```python
from build123d import *

# Parameters (mm, degrees)
EXTRUDE_2_DEPTH        = 155
CHAMFER_1_SIZE         = 2
SKETCH_5_W             = 5.5
SKETCH_5_H             = 2.5
CUT_EXTRUDE_1_DEPTH    = 156.548424936
CUT_EXTRUDE_2_REACH    = 157.444
SKETCH_6_R             = 1.925
SKETCH_7_R             = 3.55
CUT_EXTRUDE_3_DEPTH    = 3.5
PATTERN_LINEAR_1_COUNT = 15
PATTERN_LINEAR_1_PITCH = 10
PATTERN_LINEAR_2_COUNT = 8
PATTERN_LINEAR_2_PITCH = 20


with BuildPart() as part:
    # 스케치4 → 보스-돌출2 (new body)
    with BuildSketch(Plane(origin=(0, 0, 0), x_dir=(0, 0, -1), z_dir=(1, 0, 0))):
        Polygon((0, 7.5), (0, -7.5), (-2.6, -7.5), (-5.25, -10.5), (-7.75, -8), (-7.75, 8), (-5.25, 10.5), (-2.6, 7.5), align=None)
    extrude(amount=EXTRUDE_2_DEPTH)

    # 모따기1
    chamfer_1_edges = [part.edges().sort_by_distance(p)[0] for p in [
        (0, 0, 7.75),
        (155, 0, 7.75),
    ]]
    chamfer(chamfer_1_edges, length=CHAMFER_1_SIZE)

    # 스케치5 → 컷-돌출1 (cut, symmetric)
    with BuildSketch(Plane(origin=(0, 0, 0), x_dir=(1, 0, 0), z_dir=(0, 1, 0))):
        with Locations((7.3, -6.5)):
            Rectangle(SKETCH_5_W, SKETCH_5_H)
    cut_extrude_1 = extrude(amount=CUT_EXTRUDE_1_DEPTH, both=True, mode=Mode.SUBTRACT)

    # 스케치6 → 컷-돌출2 (cut, up to next)
    with BuildSketch(Plane.XY.offset(5.25), mode=Mode.PRIVATE) as cut_extrude_2_sk1:
        with Locations((7.3, 0)):
            Circle(SKETCH_6_R)
    cut_extrude_2_tool1 = extrude(cut_extrude_2_sk1.sketch, amount=-CUT_EXTRUDE_2_REACH, mode=Mode.PRIVATE) & part.part
    cut_extrude_2 = cut_extrude_2_tool1.solids().sort_by_distance((7.3, 0, 5.25))[0]
    add(cut_extrude_2, mode=Mode.SUBTRACT)

    # 스케치7 → 컷-돌출3 (cut)
    with BuildSketch(Plane.XY.offset(7.75)):
        with Locations((7.3, 0)):
            Circle(SKETCH_7_R)
    cut_extrude_3 = extrude(amount=-CUT_EXTRUDE_3_DEPTH, mode=Mode.SUBTRACT)

    # 선형 패턴1: 컷-돌출1 ×15
    with Locations(*[(i * PATTERN_LINEAR_1_PITCH, 0, 0) for i in range(1, PATTERN_LINEAR_1_COUNT)]):
        add(cut_extrude_1, mode=Mode.SUBTRACT)

    # 선형 패턴2: 컷-돌출2, 컷-돌출3 ×8
    with Locations(*[(i * PATTERN_LINEAR_2_PITCH, 0, 0) for i in range(1, PATTERN_LINEAR_2_COUNT)]):
        add(cut_extrude_2, mode=Mode.SUBTRACT)
        add(cut_extrude_3, mode=Mode.SUBTRACT)


solid = part.part
```
The model under review builds one solid part; all positions refer to its coordinate system, in mm. A direction names the side the tool comes from. Round coordinates to 2 decimals unless told otherwise and drop trailing zeros. Loops run counter-clockwise (first coordinate to the right, second up) from the corner with the lowest first, then second, coordinate; pieces in that order, holes last. Notation, with made-up numbers: M 30.5,33.25 L 69.5,33.25 A30 ccw 69.5,64.25 Z; hole C 13,74.25 d9. An arc over 180 degrees is marked long. Answer as a JSON object with one key per item and string values.
(1) Draft analysis for pull direction X (two halves, no side actions). For faces 4 (the flat face through (40.05, 0, 7)), 5 (the flat face through (2.75, 9.23, 6.52)), 6 (the flat face through (49, -2, 4.25)), state which applies: released by +X, released by -X, zero draft, split by the parting line, or undercut.
Resolved:
{"face 4": "undercut", "face 5": "zero draft", "face 6": "undercut"}
(2) Clearance check with flat-ended pins moving along their axes: P1, Ø3, axis at x = 78, y = -3.5, coming from the +Z side; P2, Ø0.8, axis at y = 7.5, z = 6.5, coming from the -X side; P3, Ø3.5, axis at x = 107, y = -1, coming from the +Z side; P4, Ø2.5, axis at x = 67.3, y = 0, coming from the +Z side. State where each tip first meets the part, or that it passes through.
Resolved:
{"P1": "z = 5.25", "P2": "x = 0.35", "P3": "z = 4.25", "P4": "through"}
(3) To check wall thickness, follow line 1 along Z through (x, y) = (49.5, 1); line 2 along Z through (x, y) = (78.5, -1); line 3 along Y through (x, z) = (147.3, 3.15) (3 decimals). State the ranges of each line that lie inside material, in increasing order.
Resolved:
{"line 1": "0 to 4.25", "line 2": "0 to 5.25", "line 3": "-8.123 to -1.925, 1.925 to 8.123"}
(4) Take a section at A-A on x = 7.3. Give the boundary of the cut face in (y, z) (3 decimals).
Resolved:
{"outline": "M -10.5,5.25 L -7.5,2.6 L -7.5,0 L -1.925,0 L -1.925,4.25 L -3.55,4.25 L -3.55,5.25 Z; M 1.925,0 L 7.5,0 L 7.5,2.6 L 10.5,5.25 L 3.55,5.25 L 3.55,4.25 L 1.925,4.25 Z"}
(5) Tool access review of faces 1 (the cylindrical face through (48.94, -3.15, 4.86)), 2 (the flat face through (42.27, 9.23, 6.52)), 3 (the flat face through (24.55, -5, 7)): name each direction out of +Z, -Z, +X, -X, +Y, -Y from which nothing blocks a thin tool from reaching the whole face with its end or side.
Resolved:
{"face 1": "+Z", "face 2": "+Z, +X, -X, +Y", "face 3": "+Z, +Y, -Y"}
